Source: CAD feature listing. Evaluate the final solid. Frame: model axes, mm. A direction names the side the tool comes from. Give positions to 0.01 mm unless a question says otherwise; leave off trailing zeros.
```python
from build123d import *

# Parameters (mm, degrees)
SKETCH1_R              = 31.75
BOSS_EXTRUDE1_DEPTH    = 22.225
SKETCH2_R              = 13.49375
SKETCH2_R_2            = 7.9375
CUT_EXTRUDE1_DEPTH     = 1.5875
SKETCH3_OUTSIDE_W      = 84.002
SKETCH3_OUTSIDE_H      = 84.002
SKETCH3_OUTSIDE_R      = 14.3129
CUT_EXTRUDE2_DEPTH     = 7.6454
SKETCH7_OUTSIDE_W      = 84.002
SKETCH7_OUTSIDE_H      = 84.002
SKETCH7_OUTSIDE_R      = 28.575
CUT_EXTRUDE3_DEPTH     = 5.08
F_10_CLEARANCE_HOLE1_D = 6.35
CUT_EXTRUDE4_DEPTH     = 6.35
CIRPATTERN1_COUNT      = 6
SKETCH9_R              = 29.174800712
SKETCH9_R_2            = 18.6055
BOSS_EXTRUDE2_DEPTH    = 0.6
FILLET1_R              = 0.396875
SKETCH10_OUTSIDE_W     = 84.002
SKETCH10_OUTSIDE_H     = 84.002
SKETCH10_OUTSIDE_R     = 7.9375
CUT_EXTRUDE5_DEPTH     = 0.79375


with BuildPart() as part:
    # Sketch1 → Boss-Extrude1 (new body)
    with BuildSketch(Plane.XY):
        Circle(SKETCH1_R)
        Polygon((2.96960111, -5.1435), (5.939202219, 0), (2.96960111, 5.1435), (-2.96960111, 5.1435), (-5.939202219, 0), (-2.96960111, -5.1435), align=None, mode=Mode.SUBTRACT)
    extrude(amount=BOSS_EXTRUDE1_DEPTH)

    # Sketch2 → Cut-Extrude1 (cut)
    with BuildSketch(Plane(origin=(0, 0, 0), x_dir=(-1, 0, 0), z_dir=(0, 0, -1))):
        Circle(SKETCH2_R)
        Circle(SKETCH2_R_2, mode=Mode.SUBTRACT)
    extrude(amount=-CUT_EXTRUDE1_DEPTH, mode=Mode.SUBTRACT)

    # Sketch3 outside → Cut-Extrude2 (cut)
    with BuildSketch(Plane.XY.offset(22.225)):
        Rectangle(SKETCH3_OUTSIDE_W, SKETCH3_OUTSIDE_H)
        Circle(SKETCH3_OUTSIDE_R, mode=Mode.SUBTRACT)
    extrude(amount=-CUT_EXTRUDE2_DEPTH, mode=Mode.SUBTRACT)

    # Sketch7 outside → Cut-Extrude3 (cut)
    with BuildSketch(Plane.XY.offset(14.5796)):
        Rectangle(SKETCH7_OUTSIDE_W, SKETCH7_OUTSIDE_H)
        Circle(SKETCH7_OUTSIDE_R, mode=Mode.SUBTRACT)
    extrude(amount=-CUT_EXTRUDE3_DEPTH, mode=Mode.SUBTRACT)

    # #10 Clearance Hole1 (through all)
    with Locations(Plane.XY.offset(14.5796)):
        with Locations((0, 23.8125)):
            f_10_clearance_hole1 = Hole(F_10_CLEARANCE_HOLE1_D / 2)

    # Sketch8 → Cut-Extrude4 (cut)
    with BuildSketch(Plane(origin=(0, 0, 0), x_dir=(-1, 0, 0), z_dir=(0, 0, -1))):
        Polygon((3.006262852, 18.6055), (6.012525703, 23.8125), (3.006262852, 29.0195), (-3.006262852, 29.0195), (-6.012525703, 23.8125), (-3.006262852, 18.6055), align=None)
    cut_extrude4 = extrude(amount=-CUT_EXTRUDE4_DEPTH, mode=Mode.SUBTRACT)

    # CirPattern1: #10 Clearance Hole1, Cut-Extrude4 ×6 about axis
    cirpattern1_axis = Axis((0, 0, 0), (0, 0, 1))
    add([f_10_clearance_hole1.rotate(cirpattern1_axis, i * 360 / CIRPATTERN1_COUNT) for i in range(1, CIRPATTERN1_COUNT)], mode=Mode.SUBTRACT)
    add([cut_extrude4.rotate(cirpattern1_axis, i * 360 / CIRPATTERN1_COUNT) for i in range(1, CIRPATTERN1_COUNT)], mode=Mode.SUBTRACT)

    # Sketch9 → Boss-Extrude2 (add)
    with BuildSketch(Plane(origin=(0, 0, 6.35), x_dir=(-1, 0, 0), z_dir=(0, 0, -1))):
        Circle(SKETCH9_R)
        Circle(SKETCH9_R_2, mode=Mode.SUBTRACT)
    extrude(amount=-BOSS_EXTRUDE2_DEPTH)

    # Fillet1
    fillet1_edges = [part.edges().sort_by_distance(p)[0] for p in [
        (-31.75, 0, 0),
        (13.49375, 0, 0),
        (7.9375, 0, 0),
        (-31.75, 0, 9.4996),
    ]]
    fillet(fillet1_edges, radius=FILLET1_R)

    # Sketch10 outside → Cut-Extrude5 (cut)
    with BuildSketch(Plane.XY.offset(22.225)):
        Rectangle(SKETCH10_OUTSIDE_W, SKETCH10_OUTSIDE_H)
        with Locations(Location((0, 0, 0), (0, 0, 180))):
            Circle(SKETCH10_OUTSIDE_R, mode=Mode.SUBTRACT)
    extrude(amount=-CUT_EXTRUDE5_DEPTH, mode=Mode.SUBTRACT)


solid = part.part
```
1. Access query for faces 1 (the flat face through (0, 18.606, 3)), 2 (the flat face through (-21, -12, 6.95)), 3 (the flat face through (-4.434, 2.608, 10.957)). Directions: +Z, -Z, +X, -X, +Y, -Y. A direction counts if a zero-diameter tool reaches every point of the face in a straight line with its end or side. Return the directions, or none.
2. Section query A-A (z = 8). Give the number of separate pieces and of enclosed holes in the cut face, plus the area to 3 significant figures.
3. Pin query (flat end, axial travel): P1, Ø3, axis at x = 21.5, z = 2.5, coming from the -Y side; P2, Ø5, axis at x = -2.5, z = 6.5, coming from the +Y side; P3, Ø3, axis at x = 21.5, z = 2, coming from the +Y side. Return the tip coordinate at first contact, or that it passes through.
4. Line query: probe 1 along Y at (x, z) = (0, 10.25) (1 decimal); probe 2 along Y at (x, z) = (2, 1.75); probe 3 along Z at (x, y) = (11.5, -4). Output: solid intervals per line, ascending.
5. Pull-direction query (X, two-part tool) for faces 4 (the flat face through (5, -2, 22.225)), 5 (the flat face through (-16.13, -9.27, 3.13)); classes: pulls with the +X half, pulls with the -X half, needs draft (parallel to the pull), parting line crosses it, or undercut.
The answers:
1. face 1: -Z
1. face 2: +Z
1. face 3: +Z, -Z
2. separate pieces: 1
2. enclosed holes: 7
2. area: 2,890 mm2
3. P1: stops at y = -24.66
3. P2: stops at y = 31.75
3. P3: stops at y = 24.66
4. probe 1: y = -28.6 to -27, -20.6 to -5.1, 5.1 to 20.6, 27 to 28.6
4. probe 2: y = -31.69 to -29.02, -18.61 to -5.14, 5.14 to 18.61, 29.02 to 31.69
4. probe 3: z = 1.59 to 21.43
5. face 4: needs draft
5. face 5: undercut
